Design review of the part built by this model. Coordinates are the model's own, in mm. Face numbers are marked on the shaded views. Round coordinates to 2 decimals unless told otherwise and drop trailing zeros. Loops run counter-clockwise (first coordinate to the right, second up) from the corner with the lowest first, then second, coordinate; pieces in that order, holes last. Notation, with made-up numbers: M -28.75,6.25 L 15.25,6.25 A31 ccw 15.25,37.25 Z; hole C -34,-39.5 d6. An arc over 180 degrees is marked long. Use a Markdown table: item, result.
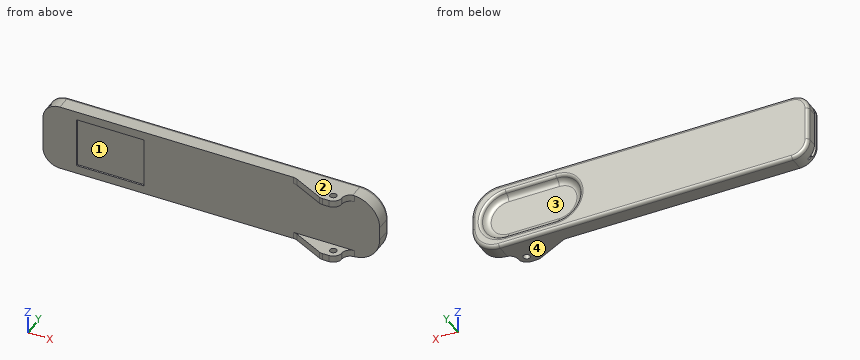
from build123d import *

# Parameters (mm, degrees)
BOSS_EXTRUDE1_DEPTH     = 5
CUT_EXTRUDE2_DEPTH      = 2
FILLET1_R               = 2
FILLET2_R               = 1
SKETCH8_W               = 18
SKETCH8_H               = 0.5
SKETCH8_W_2             = 16
CUT_EXTRUDE3_DEPTH      = 50
FILLET3_R               = 1
SKETCH9_W               = 20
SKETCH9_H               = 15
CUT_EXTRUDE4_DEPTH      = 1
SKETCH10_W              = 15
SKETCH10_H              = 2
BOSS_EXTRUDE2_DEPTH     = 5
FILLET4_R               = 2.49
CUT_EXTRUDE5_DEPTH      = 55.083269261
CUT_EXTRUDE5_DEPTH_BACK = 55.083269261
FILLET5_R               = 2.49
CUT_EXTRUDE6_DEPTH      = 55.083269261
CUT_EXTRUDE6_DEPTH_BACK = 55.083269261
SKETCH13_R              = 1


# Some blends are built 0.0001 mm under size
with BuildPart() as part:
    # Sketch2 → Boss-Extrude1 (new body)
    with BuildSketch(Plane(origin=(0, 0, 0), x_dir=(1, 0, 0), z_dir=(0, 1, 0))):
        with BuildLine():
            Line((-45, 10), (42, 10))
            ThreePointArc((42, 10), (47.656854249, 7.656854249), (50, 2))
            Line((50, 2), (50, -2))
            ThreePointArc((50, -2), (47.656854249, -7.656854249), (42, -10))
            Line((42, -10), (-45, -10))
            ThreePointArc((-45, -10), (-48.535533906, -8.535533906), (-50, -5))
            Line((-50, -5), (-50, 5))
            ThreePointArc((-50, 5), (-48.535533906, 8.535533906), (-45, 10))
        make_face()
    extrude(amount=BOSS_EXTRUDE1_DEPTH)

    # Sketch7 → Cut-Extrude2 (cut)
    with BuildSketch(Plane(origin=(0, 5, 0), x_dir=(1, 0, 0), z_dir=(0, 1, 0))):
        with BuildLine():
            Line((25, 7.25), (40, 7.25))
            ThreePointArc((40, 7.25), (47.25, 0), (40, -7.25))
            Line((40, -7.25), (25, -7.25))
            ThreePointArc((25, -7.25), (17.75, 0), (25, 7.25))
        make_face()
    extrude(amount=-CUT_EXTRUDE2_DEPTH, mode=Mode.SUBTRACT)

    # Fillet1
    fillet1_edges = [part.edges().sort_by_distance(p)[0] for p in [
        (32.5, 3, 7.25),
        (17.75, 3, 0),
        (47.25, 3, 0),
        (32.5, 3, -7.25),
    ]]
    fillet(fillet1_edges, radius=FILLET1_R - 0.0001)  # a hair under: the kernel refuses the full size

    # Fillet2
    # the kernel refuses this fillet: 1 mm, written as the material it takes off along each edge
    with BuildSketch(Plane(origin=(25, 5, 0), x_dir=(0, 0, 1), z_dir=(1, 0, 0))) as fillet2_piece_1:
        with BuildLine():
            CenterArc((8.078456413, 1), FILLET2_R, 199.469870121, 70.53012988)
            Line((8.078456413, 0), (8.078456413, -0.1))
            Line((8.078456413, -0.1), (7.25, -0.1))
            Line((7.25, -0.1), (7.15, 0))
            ThreePointArc((7.15, 0), (7.15, 0.0001), (7.041357825, 0.633357779))
            Line((7.041357825, 0.633357779), (7.135639515, 0.66668889))
        make_face()
    revolve(axis=Axis((25, 5, 0), (0, -1, 0)), revolution_arc=180, mode=Mode.SUBTRACT)
    with BuildSketch(Plane(origin=(40, 5, 7.25), x_dir=(0, 0, 1), z_dir=(-1, 0, 0))) as fillet2_piece_2:
        with BuildLine():
            CenterArc((0.828456413, -1), FILLET2_R, 90, 70.530129879)
            Line((-0.114360485, -0.66668889), (-0.208642175, -0.633357779))
            ThreePointArc((-0.208642175, -0.633357779), (-0.1, -0.0001), (-0.1, 0))
            Line((-0.1, 0), (0, 0.1))
            Line((0, 0.1), (0.828456413, 0.1))
            Line((0.828456413, 0.1), (0.828456413, 0))
        make_face()
    extrude(amount=15, mode=Mode.SUBTRACT)
    with BuildSketch(Plane(origin=(40, 5, 0), x_dir=(0, 0, -1), z_dir=(-1, 0, 0))) as fillet2_piece_3:
        with BuildLine():
            CenterArc((8.078456413, 1), FILLET2_R, 199.469870121, 70.530129879)
            Line((7.135639515, 0.66668889), (7.041357825, 0.633357779))
            ThreePointArc((7.041357825, 0.633357779), (7.15, 0.0001), (7.15, 0))
            Line((7.15, 0), (7.25, -0.1))
            Line((7.25, -0.1), (8.078456413, -0.1))
            Line((8.078456413, -0.1), (8.078456413, 0))
        make_face()
    revolve(axis=Axis((40, 5, 0), (0, -1, 0)), revolution_arc=180, mode=Mode.SUBTRACT)
    with BuildSketch(Plane(origin=(25, 5, -7.25), x_dir=(0, -0.9856047790757024, 0.16906572527610647), z_dir=(1, 0, 0))) as fillet2_piece_4:
        with BuildLine():
            CenterArc((0.845541195, 0.985596325), FILLET2_R, 189.733502803, 70.53012988)
            Line((-0.140063584, 0.8165306), (-0.238624062, 0.799624028))
            Line((-0.238624062, 0.799624028), (-0.098560478, -0.016906573))
            Line((-0.098560478, -0.016906573), (0.016906573, -0.098560478))
            ThreePointArc((0.016906573, -0.098560478), (0.017005133, -0.098543571), (0.659514694, -0.098559633))
            Line((0.659514694, -0.098559633), (0.676426194, 0))
        make_face()
    extrude(amount=15, mode=Mode.SUBTRACT)

    # Sketch8 → Cut-Extrude3 (cut)
    with BuildSketch(Plane.ZY.offset(50)):
        with Locations((0, 1.25)):
            Rectangle(SKETCH8_W, SKETCH8_H)
        with Locations((0, 0.75)):
            Rectangle(SKETCH8_W_2, SKETCH8_H)
    extrude(amount=-CUT_EXTRUDE3_DEPTH, mode=Mode.SUBTRACT)

    # Fillet3
    fillet3_edges = [part.edges().sort_by_distance(p)[0] for p in [
        (-48.535533906, 5, 8.535533906),
        (-1.5, 5, 10),
        (47.656854249, 5, 7.656854249),
        (50, 5, 0),
        (47.656854249, 5, -7.656854249),
        (-1.5, 5, -10),
        (-48.535533906, 5, -8.535533906),
        (-50, 5, 0),
    ]]
    fillet(fillet3_edges, radius=FILLET3_R)

    # Sketch9 → Cut-Extrude4 (cut)
    with BuildSketch(Plane.XZ):
        with Locations((-30, 0)):
            Rectangle(SKETCH9_W, SKETCH9_H)
    extrude(amount=-CUT_EXTRUDE4_DEPTH, mode=Mode.SUBTRACT)

    # Sketch10 → Boss-Extrude2 (add)
    with BuildSketch(Plane.XZ):
        with Locations((32.5, 9)):
            Rectangle(SKETCH10_W, SKETCH10_H)
        with Locations((32.5, -9)):
            Rectangle(SKETCH10_W, SKETCH10_H)
    extrude(amount=BOSS_EXTRUDE2_DEPTH)

    # Fillet4
    fillet4_edges = [part.edges().sort_by_distance(p)[0] for p in [
        (40, -5, -9),
        (40, 0, -9),
        (40, -5, 9),
        (40, 0, 9),
    ]]
    fillet(fillet4_edges, radius=FILLET4_R)

    # Sketch12 → Cut-Extrude5 (cut, two sides: drawn at the far end of the back side and taken through both)
    with BuildSketch(Plane.XY.offset(10).offset(-CUT_EXTRUDE5_DEPTH_BACK)):
        Polygon((25, 0), (35, -5), (35, -11.867947074), (25, -11.867947074), align=None)
    extrude(amount=CUT_EXTRUDE5_DEPTH + CUT_EXTRUDE5_DEPTH_BACK, mode=Mode.SUBTRACT)

    # Fillet5
    fillet5_edges = [part.edges().sort_by_distance(p)[0] for p in [
        (25, 0, 9),
        (25, 0, -9),
        (35, -5, -9),
        (35, -5, 9),
    ]]
    fillet(fillet5_edges, radius=FILLET5_R)

    # Sketch13 → Cut-Extrude6 (cut, two sides: drawn at the far end of the back side and taken through both)
    with BuildSketch(Plane(origin=(0, 0, -10), x_dir=(-1, 0, 0), z_dir=(0, 0, -1)).offset(-CUT_EXTRUDE6_DEPTH_BACK)):
        with Locations((-37.5, -2.5)):
            Circle(SKETCH13_R)
    extrude(amount=CUT_EXTRUDE6_DEPTH + CUT_EXTRUDE6_DEPTH_BACK, mode=Mode.SUBTRACT)


solid = part.part
1. The part is to be moulded in two halves that separate along Z. For the marked faces 1, 2, 3 and 4, say which applies: pulls with the +Z half, pulls with the -Z half, needs draft (parallel to the pull), parting line crosses it, or undercut.
Check values:
| item | result |
|---|---|
| face 1 | undercut |
| face 2 | pulls with the +Z half |
| face 3 | undercut |
| face 4 | pulls with the -Z half |
2. Insertion check: pin 1 (1.5 mm diameter, centred on x = -35.5, z = 3.5, fed in from -Y); pin 2 (8.5 mm diameter, centred on x = 34, z = 2, fed in from +Y); pin 3 (2 mm diameter, centred on x = 38.5, z = -7.5, fed in from -Y). Each pin has a flat end and moves straight along its axis. Give the tip position at first contact, or say it passes through.
Check values:
| item | result |
|---|---|
| pin 1 | stops at y = 1.5 |
| pin 2 | stops at y = 3.27 |
| pin 3 | stops at y = -5 |
3. Take a section at B-B on x = 2. Give the boundary of the cut face in (y, z).
Check values:
| item | result |
|---|---|
| outline | M 0,-10 L 4,-10 A1 ccw 5,-9 L 5,9 A1 ccw 4,10 L 0,10 Z |
4. Take a section at A-A on z = 0. Give the boundary of the cut face in (x, y), and give its area (3 significant figures).
Check values:
| item | result |
|---|---|
| outline | M -50,0 L -40,0 L -40,0.5 L -50,0.5 Z; M -50,1.5 L 0,1.5 L 0,0.5 L -20,0.5 L -20,0 L 50,0 L 50,4 A1 ccw 49,5 L 48.08,5 A1 ccw 47.14,4.33 A2 cw 45.25,3 L 19.75,3 A2 cw 17.86,4.33 A1 ccw 16.92,5 L -49,5 A1 ccw -50,4 Z |
| area | 382 mm² |
5. Wall thickness on line 1 along Y through (x, z) = (-23, 8.25); line 2 along Y through (x, z) = (37.5, -9.05); line 3 along Z through (x, y) = (28.5, -0.5): over which ranges is each line inside the solid? List them lowest first. Write a range as from..to.
Check values:
| item | result |
|---|---|
| line 1 | y = 0..1, 1.5..5 |
| line 2 | y = -5..-3.5, -1.5..5 |
| line 3 | z = -10..-8, 8..10 |
